Geometry: final body of the model. Coordinates: model frame, mm. A direction names the side the tool comes from. Give positions to 0.01 mm unless a question says otherwise; leave off trailing zeros. Write each loop counter-clockwise with the first axis right and the second up, starting at its lowest first coordinate (ties: lowest second). Pieces come first, ordered by that corner, then holes.
Q1. Reachability of faces 1 (the face through (13, 19, 0)), 2 (the face through (0, 28, 3)), 3 (the face through (11, -12.5, 5)), 4 (the face through (1, 24.4, 3)) from +Z, -Z, +X, -X, +Y, -Y: full face, straight path, thin tool, end or side. Return the list, or none.
Q2. Cut plane C-C on y = -4.5. Return the cut outline in (x, z), plus the area to 3 significant figures.
Q3. Cut plane D-D on x = 3. Return the cut outline in (y, z), plus the area to 3 significant figures.
Q4. Line query: L1, parallel to X at y = -0.5, z = -0.75; L2, parallel to X at y = 7.5, z = 3.25; L3, parallel to Y at x = 12, z = 5.25. Output: solid intervals per line, ascending.
Q5. Draft query along X for faces 5 (the face through (-16.5, 12, 3)), 6 (the face through (-11, -12.5, 3)), 7 (the face through (-10, 8, -1)). Return one class per face: pulls with the +X half, pulls with the -X half, needs draft (parallel to the pull), parting line crosses it, or undercut.
Q6. Cut plane A-A on z = 6. Return the cut outline in (x, y).
Q7. Pin query (flat end, axial travel): pin 1 (1.5 mm diameter, centred on x = -4.5, y = 22.5, fed in from +Z); pin 2 (1.5 mm diameter, centred on x = 2.5, z = 2, fed in from -Y). Return the tip coordinate at first contact, or that it passes through.
Q8. Cut plane B-B on y = 17. Return the cut outline in (x, z).
```python
from build123d import *

# Parameters (mm, degrees)
ESBO_O1_W                = 7.5
ESBO_O1_H                = 5
ESBO_O1_H_2              = 19
ESBO_O1_W_2              = 6
ESBO_O1_H_3              = 6
ESBO_O1_H_4              = 1.5
ESBO_O1_H_5              = 1
ESBO_O1_W_3              = 1.5
ESBO_O1_H_6              = 8.5
RESSALTO_EXTRUS_O5_DEPTH = 1.6
RESSALTO_EXTRUS_O6_DEPTH = 7
RESSALTO_EXTRUS_O7_DEPTH = 3


with BuildPart() as part:
    # Esbo_o1 → Ressalto-extrus_o5 (new body)
    with BuildSketch(Plane.XY):
        Polygon((-16.5, -4), (-15, -4), (-15, 0), (-15, 26.5), (0, 26.5), (15, 26.5), (15, 0), (15, -12.5), (6, -12.5), (6, -14), (16.5, -14), (16.5, 0), (16.5, 28), (0, 28), (-16.5, 28), (-16.5, 0), align=None)
        Polygon((13.5, 25), (13.5, 19), (13.5, 0), (13.5, -4), (13.5, -11), (6, -11), (6, -12.5), (15, -12.5), (15, 0), (15, 26.5), (0, 26.5), (-15, 26.5), (-15, 0), (-15, -4), (-13.5, -4), (-13.5, 0), (-13.5, 19), (-13.5, 25), (0, 25), align=None)
        Polygon((-7.5, 24), (0, 24), (7.5, 24), (12.5, 24), (12.5, 19), (13.5, 19), (13.5, 25), (0, 25), (-13.5, 25), (-13.5, 19), (-12.5, 19), (-12.5, 24), align=None)
        Polygon((-10, 0), (-7.5, 0), (-7.5, 19), (-7.5, 24), (-12.5, 24), (-12.5, 19), (-10, 19), align=None)
        with Locations((-3.75, 21.5)):
            Rectangle(ESBO_O1_W, ESBO_O1_H)
        with Locations((3.75, 21.5)):
            Rectangle(ESBO_O1_W, ESBO_O1_H)
        Polygon((7.5, 19), (7.5, 0), (10, 0), (10, 19), (12.5, 19), (12.5, 24), (7.5, 24), align=None)
        with Locations((3.75, 9.5)):
            Rectangle(ESBO_O1_W, ESBO_O1_H_2)
        with Locations((-3.75, 9.5)):
            Rectangle(ESBO_O1_W, ESBO_O1_H_2)
        Polygon((7.5, 0), (0, 0), (-7.5, 0), (-10, 0), (-10, -4), (-6, -4), (0, -4), (6, -4), (10, -4), (10, 0), align=None)
        Polygon((-6, -4), (-10, -4), (-12.5, -4), (-12.5, -10), (-6, -10), align=None)
        with Locations((-3, -7)):
            Rectangle(ESBO_O1_W_2, ESBO_O1_H_3)
        with Locations((3, -7)):
            Rectangle(ESBO_O1_W_2, ESBO_O1_H_3)
        Polygon((12.5, -4), (10, -4), (6, -4), (6, -10), (12.5, -10), align=None)
        with Locations((3, -11.75)):
            Rectangle(ESBO_O1_W_2, ESBO_O1_H_4)
        Polygon((13.5, -4), (12.5, -4), (12.5, -10), (6, -10), (6, -11), (13.5, -11), align=None)
        with Locations((3, -10.5)):
            Rectangle(ESBO_O1_W_2, ESBO_O1_H_5)
        with Locations((-3, -10.5)):
            Rectangle(ESBO_O1_W_2, ESBO_O1_H_5)
        with Locations((-3, -11.75)):
            Rectangle(ESBO_O1_W_2, ESBO_O1_H_4)
        Polygon((-13.5, -11), (-13.5, -4), (-15, -4), (-15, -12.5), (-6, -12.5), (-6, -11), align=None)
        Polygon((-12.5, -10), (-12.5, -4), (-13.5, -4), (-13.5, -11), (-6, -11), (-6, -10), align=None)
        with Locations((-15.75, -8.25)):
            Rectangle(ESBO_O1_W_3, ESBO_O1_H_6)
        Polygon((-6, -14), (-6, -12.5), (-15, -12.5), (-16.5, -12.5), (-16.5, -14), align=None)
        Polygon((6, -14), (6, -12.5), (0, -12.5), (-6, -12.5), (-6, -14), align=None)
    extrude(amount=-RESSALTO_EXTRUS_O5_DEPTH)

    # Esbo_o1_4 → Ressalto-extrus_o6 (add)
    with BuildSketch(Plane.XY):
        Polygon((-16.5, -4), (-15, -4), (-15, 0), (-15, 26.5), (0, 26.5), (15, 26.5), (15, 0), (15, -12.5), (6, -12.5), (6, -14), (16.5, -14), (16.5, 0), (16.5, 28), (0, 28), (-16.5, 28), (-16.5, 0), align=None)
        Polygon((-6, -14), (-6, -12.5), (-15, -12.5), (-16.5, -12.5), (-16.5, -14), align=None)
    extrude(amount=RESSALTO_EXTRUS_O6_DEPTH)

    # Esbo_o1_5 → Ressalto-extrus_o7 (add)
    with BuildSketch(Plane.XY):
        Polygon((13.5, 25), (13.5, 19), (13.5, 0), (13.5, -4), (13.5, -11), (6, -11), (6, -12.5), (15, -12.5), (15, 0), (15, 26.5), (0, 26.5), (-15, 26.5), (-15, 0), (-15, -4), (-13.5, -4), (-13.5, 0), (-13.5, 19), (-13.5, 25), (0, 25), align=None)
        Polygon((-7.5, 24), (0, 24), (7.5, 24), (12.5, 24), (12.5, 19), (13.5, 19), (13.5, 25), (0, 25), (-13.5, 25), (-13.5, 19), (-12.5, 19), (-12.5, 24), align=None)
    extrude(amount=RESSALTO_EXTRUS_O7_DEPTH)


solid = part.part
```
Data:
1. face 1: +Z, -Z
1. face 2: +Z, -Z, +X, -X, +Y
1. face 3: +Z, -X
1. face 4: +Z
2. outline: (-16.5, -1.6) - (16.5, -1.6) - (16.5, 7) - (15, 7) - (15, 3) - (13.5, 3) - (13.5, 0) - (-16.5, 0) - close
2. area: 67.8 mm2
3. outline: (-14, -1.6) - (28, -1.6) - (28, 7) - (26.5, 7) - (26.5, 3) - (24, 3) - (24, 0) - (-14, 0) - close
3. area: 85.2 mm2
4. L1: x = -16.5 to -13.5, -10 to 10, 13.5 to 16.5
4. L2: x = -16.5 to -15, 15 to 16.5
4. L3: y = -14 to -12.5, 26.5 to 28
5. face 5: pulls with the -X half
5. face 6: needs draft
5. face 7: undercut
6. outline: (-16.5, -14) - (-6, -14) - (-6, -12.5) - (-16.5, -12.5) - close; (-16.5, -4) - (-15, -4) - (-15, 26.5) - (15, 26.5) - (15, -12.5) - (6, -12.5) - (6, -14) - (16.5, -14) - (16.5, 28) - (-16.5, 28) - close
7. pin 1: stops at z = 0
7. pin 2: stops at y = 24
8. outline: (-16.5, -1.6) - (-13.5, -1.6) - (-13.5, 3) - (-15, 3) - (-15, 7) - (-16.5, 7) - close; (-10, -1.6) - (10, -1.6) - (10, 0) - (-10, 0) - close; (13.5, -1.6) - (16.5, -1.6) - (16.5, 7) - (15, 7) - (15, 3) - (13.5, 3) - close
